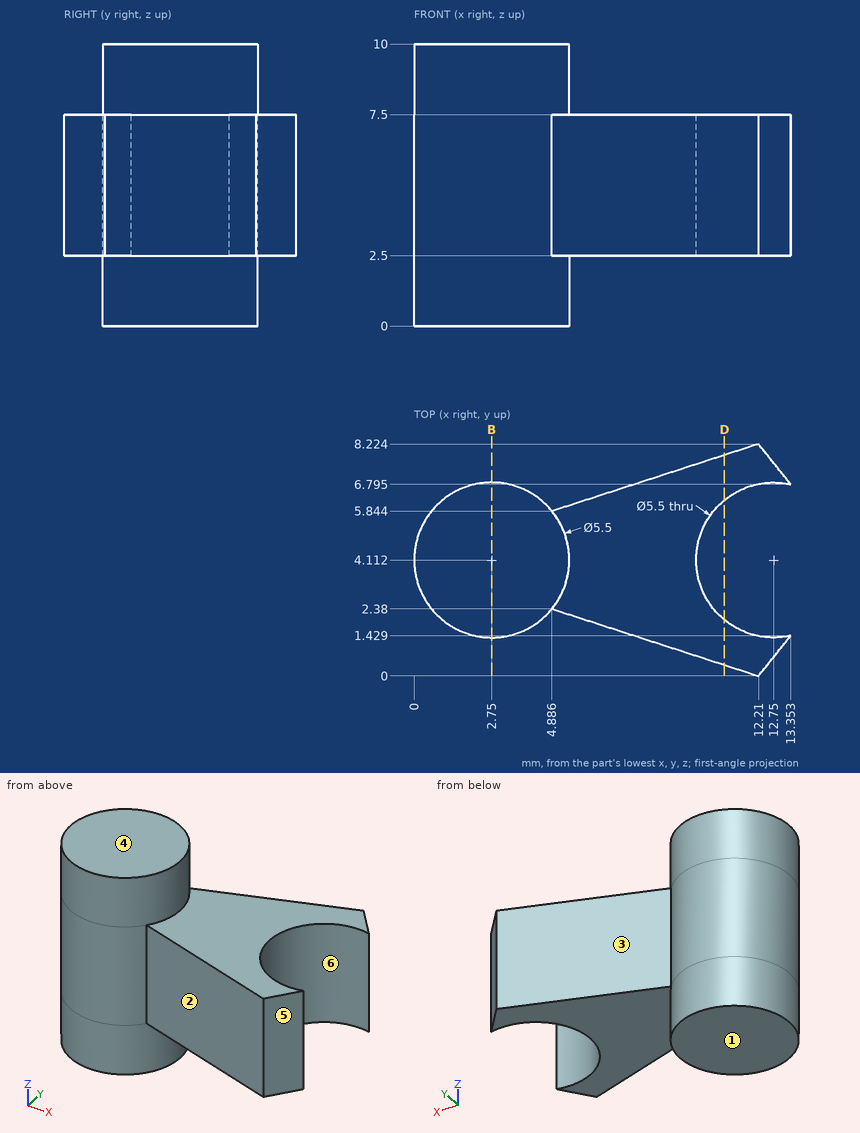
Part print with two shaded views. Sizes in mm from the minimum x, y, z corner. A direction names the side the tool comes from. Round coordinates to 2 decimals unless told otherwise and drop trailing zeros. Loops run counter-clockwise (first coordinate to the right, second up) from the corner with the lowest first, then second, coordinate; pieces in that order, holes last.
Item 1: Two-plate mould, pull along X, no slides. Class the marked faces 4, 5 and 6: released by +X, released by -X, zero draft, split by the parting line, or undercut.
Item 2: Saw through at B-B (x = 2.75). List the corners of the cut face in (y, z), then the cut area to 3 significant figures.
Item 3: Pin check, flat tips, straight feed: P1, Ø6, axis at x = 2, z = 5.5, coming from the -Y side; P2, Ø4, axis at x = 10, y = 3, coming from the -Z side; P3, Ø5, axis at x = 6, z = 1.5, coming from the -Y side. Stop position of each tip, or through.
Item 4: Drill centre lines: line 1 along Z through (x, y) = (8.5, 3); line 2 along Y through (x, z) = (5.25, 8.25) (1 decimal); line 3 along Y through (x, z) = (2.25, 3.75). Where is each one in solid material? Low to high.
Item 5: Saw through at D-D (x = 11). List the corners of the cut face in (y, z), then the cut area to 3 significant figures.
Item 6: Which spindle directions (+Z, -Z, +X, -X, +Y, -Y) get a long thin tool onto all of the face, cutting with end or side? Do the marked faces 1, 2 and 3. Say none if no direction does.
Worked answers:
1. face 4: zero draft
1. face 5: released by +X
1. face 6: undercut
2. outline: (1.36, 0) - (6.86, 0) - (6.86, 10) - (1.36, 10) - close
2. area: 55.0 mm2
3. P1: stops at y = 1.36
3. P2: stops at z = 2.5
3. P3: stops at y = 1.27
4. line 1: z = 2.5 to 7.5
4. line 2: y = 3 to 5.3
4. line 3: y = 1.41 to 6.82
5. outline: (0.39, 2.5) - (1.99, 2.5) - (1.99, 7.5) - (0.39, 7.5) - close; (6.23, 2.5) - (7.83, 2.5) - (7.83, 7.5) - (6.23, 7.5) - close
5. area: 16.0 mm2
6. face 1: -Z, +X, -X, +Y, -Y
6. face 2: +Z, -Z, -Y
6. face 3: +Z, -Z, +Y
